Read the model definition and answer for the solid it produces. Units are mm, in the model's axes. A direction names the side the tool comes from. Coordinates: 2 decimals unless noted, no trailing zeros. Loops run counter-clockwise (first coordinate to the right, second up) from the corner with the lowest first, then second, coordinate; pieces in that order, holes last. Notation, with made-up numbers: (51, 85) - (90, 85) arc R21 ccw to (90, 121) - close; hole circle Ø3 at (55.25, -21). An arc over 180 degrees is marked (long way). One line per item, written item: value. Start each with the question number.
from build123d import *

# Parameters (mm, degrees)
F1_W      = 40
F1_H      = 35
F2_DEPTH  = 70
F3_DEPTH  = 30
F5_DEPTH  = 103
F6_R      = 20
F8_DEPTH  = 28
F10_DEPTH = 140
F12_DEPTH = 1016
F13_R     = 20
F15_DEPTH = 80
F17_DEPTH = 396


with BuildPart() as f2:
    # F1 (on face) → F2 (new body)
    with BuildSketch(Plane.XY):
        with Locations((-47.2459378839, 1.8207169324)):
            Rectangle(F1_W, F1_H)
    extrude(amount=F2_DEPTH)

    # F0 (on Top) → F3 (join)
    with BuildSketch(Plane.XY):
        Polygon((172.7540621161, 134.3207169324), (-67.2459378839, 134.3207169324), (-67.2459378839, -15.6792830676), (-27.2459378839, -15.6792830676), (-27.2459378839, 19.3207169324), (52.7540621161, 19.3207169324), (52.7540621161, -15.6792830676), (172.7540621161, -15.6792830676), align=None)
    extrude(amount=F3_DEPTH)

    # F4 (on face) → F5 (cut)
    with BuildSketch(Plane.YZ.offset(-27.2459378839)):
        Polygon((-15.6792830676, 70), (-15.6792830676, 30), (19.3207169324, 70), align=None)
    extrude(amount=-F5_DEPTH, mode=Mode.SUBTRACT)

    # F6
    f6_edges = [f2.edges().sort_by_distance(p)[0] for p in [
        (172.754062, -15.679283, 15),
        (172.754062, 134.320717, 15),
    ]]
    fillet(f6_edges, radius=F6_R)

    # F7 (on face) → F8 (cut)
    with BuildSketch(Plane(origin=(0, 19.3207169324, 0), x_dir=(-1, 0, 0), z_dir=(0, 1, 0))):
        with BuildLine():
            ThreePointArc((57.2459378839, 50), (54.3170056957, 57.0710678119), (47.2459378839, 60))
            Line((47.2459378839, 60), (47.2459378839, 40))
            ThreePointArc((47.2459378839, 40), (54.3170056957, 42.9289321881), (57.2459378839, 50))
        make_face()
        with BuildLine():
            Line((47.2459378839, 40), (47.2459378839, 60))
            ThreePointArc((47.2459378839, 60), (37.2459378839, 50), (47.2459378839, 40))
        make_face()
    extrude(amount=-F8_DEPTH, mode=Mode.SUBTRACT)

    # F9 (on face) → F10 (join)
    with BuildSketch(Plane(origin=(0, 0, 0), x_dir=(1, 0, 0), z_dir=(0, 0, -1))):
        Polygon((52.7540621161, -134.3207169324), (52.7540621161, -19.3207169324), (-27.2459378839, -19.3207169324), (-67.2459378839, -19.3207169324), (-67.2459378839, -134.3207169324), align=None)
    extrude(amount=-F10_DEPTH)

    # F11 (on face) → F12 (cut)
    with BuildSketch(Plane.XZ.offset(-19.3207169324)):
        Polygon((52.7540621161, 140), (2.7540621161, 140), (52.7540621161, 30), align=None)
    extrude(amount=-F12_DEPTH, mode=Mode.SUBTRACT)

    # F13
    f13_edges = [f2.edges().sort_by_distance(p)[0] for p in [
        (52.754062, 76.820717, 30),
    ]]
    fillet(f13_edges, radius=F13_R)

    # F14 (on face) → F15 (cut)
    with BuildSketch(Plane.XY.offset(30)):
        with BuildLine():
            ThreePointArc((94.1931948194, 59.3207169324), (119.1931948194, 34.3207169324), (144.1931948194, 59.3207169324))
            Line((144.1931948194, 59.3207169324), (94.1931948194, 59.3207169324))
        make_face()
        with BuildLine():
            Line((94.1931948194, 59.3207169324), (144.1931948194, 59.3207169324))
            ThreePointArc((144.1931948194, 59.3207169324), (119.1931948194, 84.3207169324), (94.1931948194, 59.3207169324))
        make_face()
    extrude(amount=-F15_DEPTH, mode=Mode.SUBTRACT)

    # F16 (on face) → F17 (cut)
    with BuildSketch(Plane(origin=(-67.2459378839, 0, 0), x_dir=(0, -1, 0), z_dir=(-1, 0, 0))):
        with BuildLine():
            ThreePointArc((-76.8207169324, 135), (-94.4983864621, 92.3223304703), (-51.8207169324, 110))
            ThreePointArc((-51.8207169324, 110), (-59.1430474028, 127.6776695297), (-76.8207169324, 135))
        make_face()
    extrude(amount=-F17_DEPTH, mode=Mode.SUBTRACT)


solid = f2.part
1) Section D-D, the plane y = 62.5 is taken. Determine the outline of the cut face in (x, z) (3 decimals), and give its area (3 significant figures).
2) Determine the mould class of faces 1 (the cylindrical face through (166.74, 128.62, 15.21)), 2 (the flat face through (-38.08, -2.31, 45.28)), 3 (the flat face through (-47, 19.321, 50)) for opening direction X: released by +X, released by -X, zero draft, split by the parting line, or undercut.
3) Section C-C, the plane x = 129.5 is taken. Determine the outline of the cut face in (y, z), and give its area (3 significant figures).
4) Straight lines are drawn through the part: L1, parallel to Y at x = -44, z = 110; L2, parallel to Z at x = 69, y = 82.5; L3, parallel to Z at x = 2.5, y = 82. For each, find the intervals that lie inside material, in ascending order.
5) Section B-B, the plane y = 44 is taken. Determine the outline of the cut face in (x, z) (3 decimals), and give its area (3 significant figures).
6) Flat-ended cylindrical pins translate along their axes: P1, Ø10, axis at y = 46.5, z = 96.5, coming from the +X side; P2, Ø10, axis at x = -44.5, z = 51.5, coming from the -Y side; P3, Ø12, axis at y = 118.5, z = 41.5, coming from the +X side. Find the tip coordinate at first contact, or state that the pin passes through.
7) Section A-A, the plane z = 104 is taken. Determine the outline of the cut face in (x, y), and give its area (3 significant figures).
8) For faces 4 (the flat face through (51, 60, 0)), 5 (the flat face through (52.754, 2, 15)), determine the directions among +Z, -Z, +X, -X, +Y, -Y from which every point of the face is accessible in a straight line to the end or side of a thin tool.
Answer below:
1. outline: (-67.246, 0) - (94.396, 0) - (94.396, 30) - (65.632, 30) arc R20 cw to (47.425, 41.724) - (25.705, 89.508) - (-67.246, 89.508) - close; (-67.246, 130.492) - (7.076, 130.492) - (2.754, 140) - (-67.246, 140) - close; (143.99, 0) - (172.754, 0) - (172.754, 30) - (143.99, 30) - close
1. area: 12,800 mm2
2. face 1: released by +X
2. face 2: zero draft
2. face 3: undercut
3. outline: (-15.68, 0) - (36.54, 0) - (36.54, 30) - (-15.68, 30) - close; (82.1, 0) - (134.32, 0) - (134.32, 30) - (82.1, 30) - close
3. area: 3,130 mm2
4. L1: 19.32 to 51.82, 101.82 to 134.32
4. L2: 0 to 30
4. L3: 0 to 85.54, 134.46 to 140
5. outline: (-67.246, 0) - (99.438, 0) - (99.438, 30) - (65.632, 30) arc R20 cw to (47.425, 41.724) - (2.754, 140) - (-67.246, 140) - close; (138.949, 0) - (172.754, 0) - (172.754, 30) - (138.949, 30) - close
5. area: 16,500 mm2
6. P1: x = 24.8
6. P2: y = 19.32
6. P3: x = 51.86
7. outline: (-67.25, 19.32) - (19.12, 19.32) - (19.12, 52.55) - (-67.25, 52.55) - close; (-67.25, 101.09) - (19.12, 101.09) - (19.12, 134.32) - (-67.25, 134.32) - close
7. area: 5,740 mm2
8. face 4: -Z, +X, -X, +Y, -Y
8. face 5: +Z, -Z, -Y
